Could you check a few things on this model? Use its own coordinates, in mm. Face numbers are marked on the shaded views. Round coordinates to 2 decimals unless told otherwise and drop trailing zeros. Loops run counter-clockwise (first coordinate to the right, second up) from the corner with the lowest first, then second, coordinate; pieces in that order, holes last. Notation, with made-up numbers: (4, -23.75) -> (8, -23.75) arc R14 cw to (8, -4.75) -> close; hole circle Ø11 at (-1, 8.25). An arc over 180 degrees is marked (long way). One line per item, written item: value.
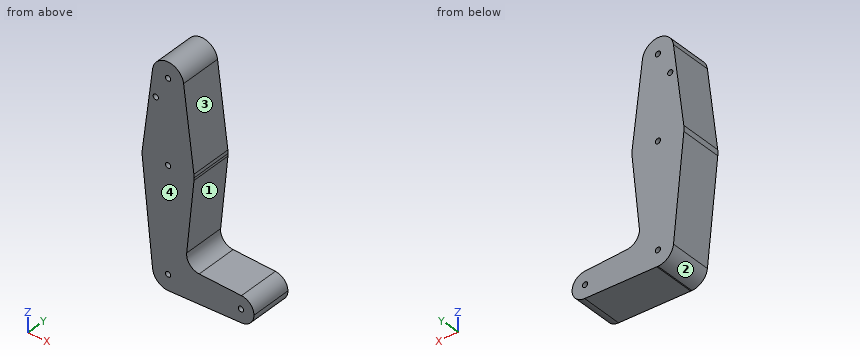
```python
from build123d import *

# Parameters (mm, degrees)
F0_R     = 1.5875
F1_DEPTH = 25.4


with BuildPart() as f1:
    # F0 (on Front) → F1 (new body)
    with BuildSketch(Plane.XZ):
        with BuildLine():
            ThreePointArc((-9.450293, 115.490625), (-0.596483, 104.793695), (9.525, 114.3))
            ThreePointArc((9.525, 114.3), (9.506305, 114.896483), (9.450293, 115.490625))
            ThreePointArc((9.450293, 115.490625), (0, 123.825), (-9.450293, 115.490625))
        make_face()
        with Locations((0, 114.3)):
            Circle(F0_R, mode=Mode.SUBTRACT)
        with BuildLine():
            ThreePointArc((9.450293, 115.490625), (9.506305, 114.896483), (9.525, 114.3))
            ThreePointArc((9.525, 114.3), (-0.596483, 104.793695), (-9.450293, 115.490625))
            Line((-9.450293, 115.490625), (-15.750488, 65.484375))
            ThreePointArc((-15.750488, 65.484375), (0, 79.375), (15.750488, 65.484375))
            Line((15.750488, 65.484375), (9.450293, 115.490625))
        make_face()
        with Locations((-7.514715, 100.0252)):
            Circle(F0_R, mode=Mode.SUBTRACT)
        with BuildLine():
            ThreePointArc((15.875, 63.5), (15.843841, 64.494139), (15.750488, 65.484375))
            ThreePointArc((15.750488, 65.484375), (0, 79.375), (-15.750488, 65.484375))
            ThreePointArc((-15.750488, 65.484375), (-15.873744, 63.699705), (-15.795426, 61.9125))
            ThreePointArc((-15.795426, 61.9125), (0, 47.625), (15.795426, 61.9125))
            ThreePointArc((15.795426, 61.9125), (15.855094, 62.705253), (15.875, 63.5))
        make_face()
        with Locations((0, 63.5)):
            Circle(F0_R, mode=Mode.SUBTRACT)
        with BuildLine():
            ThreePointArc((15.795426, 61.9125), (0, 47.625), (-15.795426, 61.9125))
            Line((-15.795426, 61.9125), (-9.477255, -0.9525))
            ThreePointArc((-9.477255, -0.9525), (-7.063929, 6.389564), (0, 9.525))
            ThreePointArc((0, 9.525), (0.338886, 9.51897), (0.677344, 9.500886))
            ThreePointArc((0.677344, 9.500886), (6.970557, 6.491299), (9.525, 0))
            ThreePointArc((9.525, 0), (9.513056, -0.476848), (9.477255, -0.9525))
            ThreePointArc((9.477255, -0.9525), (6.636844, -6.832125), (0.677344, -9.500886))
            Line((0.677344, -9.500886), (44.732405, -7.932475))
            ThreePointArc((44.732405, -7.932475), (36.5125, 0), (44.732405, 7.932475))
            Line((44.732405, 7.932475), (18.968328, 8.849706))
            ThreePointArc((18.968328, 8.849706), (13.261204, 11.567463), (11.340836, 17.589892))
            Line((11.340836, 17.589892), (15.795426, 61.9125))
        make_face()
        with BuildLine():
            ThreePointArc((0, 9.525), (-7.063929, 6.389564), (-9.477255, -0.9525))
            ThreePointArc((-9.477255, -0.9525), (-6.389564, -7.063929), (0, -9.525))
            Line((0, -9.525), (0.677344, -9.500886))
            ThreePointArc((0.677344, -9.500886), (6.636844, -6.832125), (9.477255, -0.9525))
            ThreePointArc((9.477255, -0.9525), (9.513056, -0.476848), (9.525, 0))
            ThreePointArc((9.525, 0), (6.970557, 6.491299), (0.677344, 9.500886))
            Line((0.677344, 9.500886), (0, 9.525))
        make_face()
        Circle(F0_R, mode=Mode.SUBTRACT)
        with BuildLine():
            Line((0.677344, -9.500886), (0, -9.525))
            ThreePointArc((0, -9.525), (0.338886, -9.51897), (0.677344, -9.500886))
        make_face()
        with BuildLine():
            ThreePointArc((52.3875, 0), (50.161633, 5.51191), (44.732405, 7.932475))
            ThreePointArc((44.732405, 7.932475), (36.5125, 0), (44.732405, -7.932475))
            ThreePointArc((44.732405, -7.932475), (50.161633, -5.51191), (52.3875, 0))
        make_face()
        with Locations((44.45, 0)):
            Circle(F0_R, mode=Mode.SUBTRACT)
    extrude(amount=F1_DEPTH)


solid = f1.part
```
(1) Imagine slicing it at C-C on z = 75. Write out the boundary of the cut face in (x, y).
Results below:
outline: (-14.55, -25.4) -> (14.55, -25.4) -> (14.55, 0) -> (-14.55, 0) -> close
(2) Imagine slicing it at B-B on x = 48.5. Write out the boundary of the cut face in (y, z).
Results below:
outline: (-25.4, -6.83) -> (0, -6.83) -> (0, 6.83) -> (-25.4, 6.83) -> close
(3) For pin 1 Ø1 at (y, z) = (-19, 78) entering from -X; pin 2 Ø10 at (y, z) = (-3, 58) entering from +X; pin 3 Ø5 at (x, y) = (42, -3) entering from +Z, each with a flat end and sliding along its axis, tell me the tip position at first contact or that it passes through.
Results below:
pin 1: stops at x = -14.24
pin 2: stops at x = 15.87
pin 3: stops at z = 8.12
(4) Imagine slicing it at A-A on y = -15. Give the number of separate pieces and of enclosed holes in the cut face, then the cut area to 3 significant figures.
Results below:
separate pieces: 1
enclosed holes: 6
area: 3,890 mm²
(5) Please list where these lines run through material, in increasing order: L1, parallel to X at y = -1.5, z = -1; L2, parallel to X at y = -7.25, z = 114.3; L3, parallel to Z at x = 28.5, y = -10.
Results below:
L1: x = -9.47 to -1.23, 1.23 to 43.22, 45.68 to 52.32
L2: x = -9.6 to -1.59, 1.59 to 9.6
L3: z = -8.51 to 8.51
(6) We'd pull the mould along Z, two halves only. Please class the marked faces 1, 2, 3 and 4: +Z half, -Z half, draft (parallel to the pull), parting line (faces both ways), or undercut.
Results below:
face 1: undercut
face 2: -Z half
face 3: +Z half
face 4: draft
